Autodesk Inventor part; units mm, degrees
ref_plane "YZ Plane" through (0, 0, 0) normal (1, 0, 0) x (0, 1, 0)
ref_plane "XZ Plane" through (0, 0, 0) normal (0, 1, 0) x (-1, 0, 0)
ref_plane "XY Plane" through (0, 0, 0) normal (0, 0, 1) x (1, 0, 0)
sketch "Sketch1" plane through (0, 0, 0) normal (0, 1, 0) x (-1, 0, 0)
  circle A0 centre (0, 0) radius 84.75
  dimension "d0" = 169.5
extrude "Extrusion1" add sketch "Sketch1" along normal blind 15
sketch "Sketch2" plane through (0, 0, 0) normal (0, -1, 0) x (1, 0, 0)
  circle A0 centre (0, 0) radius 76
  circle A1 centre (0, 76) radius 4
  circle A2 centre (0, -76) radius 4
  circle A3 centre (0, 76) radius 2.25
  circle A4 centre (0, -76) radius 2.25
  dimension "d3" = 152
  dimension "d4" = 8
  dimension "d5" = 8
  dimension "d6" = 4.5
  dimension "d7" = 4.5
extrude "Extrusion2" cut sketch "Sketch2" against normal through all contours A3 A0 | A0 A3 | A4 A0 | A0 A4
extrude "Extrusion3" cut sketch "Sketch2" against normal blind 12 contours A1 A0 A3 | A0 A3 A1 | A2 A0 A4 | A0 A4 A2 | A3 A0 | A0 A3 | A4 A0 | A0 A4
sketch "Sketch3" plane through (0, 0, 0) normal (0, -1, 0) x (1, 0, 0)
  circle A0 centre (0, 0) radius 84.75
  circle A1 centre (0, 0) radius 20
  circle A2 centre (0, -20) radius 4
  circle A3 centre (20, 0) radius 4
  circle A4 centre (0, 20) radius 4
  circle A5 centre (-20, 0) radius 4
  line L0 (55, 55) -> (-55, 55)
  line L1 (-55, 55) -> (-55, -55)
  line L2 (-55, -55) -> (55, -55)
  line L3 (55, -55) -> (55, 55)
  line L4 (55, 55) -> (-55, -55) construction
  line L5 (-55, 55) -> (55, -55) construction
  circle A6 centre (0, 0) radius 55
  circle A7 centre (-38.8909, -38.8909) radius 4
  circle A8 centre (38.8909, -38.8909) radius 4
  circle A9 centre (38.8909, 38.8909) radius 4
  circle A10 centre (-38.8909, 38.8909) radius 4
  dimension "d12" = 40
  dimension "d13" = 8
  dimension "d16" = 360
  dimension "d21" = 110
  dimension "d22" = 110
  dimension "d23" = 110
  dimension "d24" = 8
  dimension "d25" = 8
  dimension "d26" = 8
  dimension "d27" = 8
hole "Hole1" at (38.8909, 0, -38.8909) at (38.8909, 0, 38.8909) at (-38.8909, 0, 38.8909) at (-38.8909, 0, -38.8909) direction (0, 1, 0) diameter 6.647 depth 20 tip angle 118
sketch "Sketch4" plane through (0, 0, 0) normal (0, -1, 0) x (1, 0, 0)
  circle A0 centre (0, 0) radius 47.5
  circle A1 centre (-47.5, 0) radius 2.5
  circle A2 centre (-43.8843, -18.1775) radius 2.5
  circle A3 centre (-33.5876, -33.5876) radius 2.5
  circle A4 centre (-18.1775, -43.8843) radius 2.5
  circle A5 centre (0, -47.5) radius 2.5
  circle A6 centre (18.1775, -43.8843) radius 2.5
  circle A7 centre (33.5876, -33.5876) radius 2.5
  circle A8 centre (43.8843, -18.1775) radius 2.5
  circle A9 centre (47.5, 0) radius 2.5
  circle A10 centre (43.8843, 18.1775) radius 2.5
  circle A11 centre (33.5876, 33.5876) radius 2.5
  circle A12 centre (18.1775, 43.8843) radius 2.5
  circle A13 centre (0, 47.5) radius 2.5
  circle A14 centre (-18.1775, 43.8843) radius 2.5
  circle A15 centre (-33.5876, 33.5876) radius 2.5
  circle A16 centre (-43.8843, 18.1775) radius 2.5
  dimension "d35" = 95
  dimension "d36" = 5
  dimension "d39" = 360
hole "Hole2" at (43.8843, 0, 18.1775) at (-43.8843, 0, -18.1775) direction (0, 1, 0) diameter 5 end through all
sketch "Sketch5" plane through (0, 15, 0) normal (0, 1, 0) x (1, 0, 0)
  circle A0 centre (0, 0) radius 84.75
hole "Hole3" at (0, 15, 0) direction (0, -1, 0) diameter 10.106 depth 32.3 tip angle 118 counterbore diameter 21 counterbore depth 13
sketch "Sketch6" plane through (0, 15, 0) normal (0, 1, 0) x (1, 0, 0)
  circle A0 centre (-38.8909, -38.8909) radius 3.3235
  circle A1 centre (-38.8909, -38.8909) radius 3.3235
  circle A2 centre (-38.8909, 38.8909) radius 3.3235
  circle A3 centre (-38.8909, 38.8909) radius 3.3235
  circle A4 centre (38.8909, 38.8909) radius 3.3235
  circle A5 centre (38.8909, 38.8909) radius 3.3235
  circle A6 centre (38.8909, -38.8909) radius 3.3235
  circle A7 centre (38.8909, -38.8909) radius 3.3235
  point P0 (0, 0)
hole "Hole4" at (-38.8909, 15, 38.8909) at (-38.8909, 15, -38.8909) at (38.8909, 15, 38.8909) at (38.8909, 15, -38.8909) direction (0, -1, 0) diameter 6.647 depth 20 tip angle 118 counterbore diameter 19 counterbore depth 9
properties part number "substrate plate"
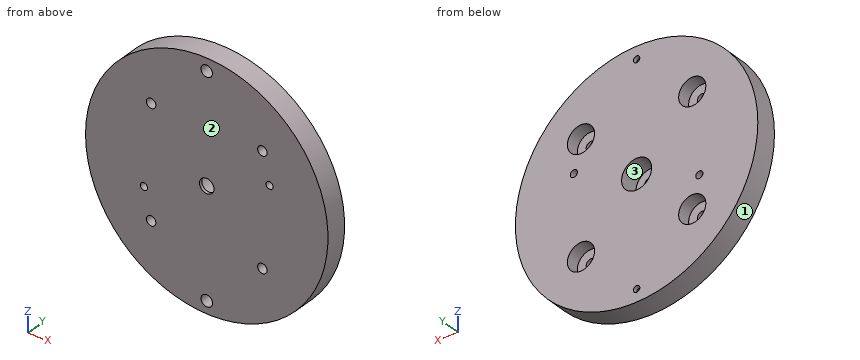
CAD build for the part. Positions are in the model's coordinates, mm. Face numbers are marked on the shaded views. Coordinates: 2 decimals unless noted, no trailing zeros. Order: outer loops, then holes, each group sorted by start corner. A loop starts at its lowest first (then second) coordinate and runs counter-clockwise, first axis right, second up. Notation, with made-up numbers: (-15.75, 2) - (0.25, 2) arc R12 cw to (0.25, 25) - close; hole circle Ø7 at (65, 69.25). An arc over 180 degrees is marked (long way). Use a Markdown table: item, result. Add a question column.
(1) Saw through at B-B (x = 0). Give the cut face in (y, z), then the cut area to 3 significant figures.
(2) Saw through at C-C (z = -76). Give the cut face in (x, y), then the cut area to 3 significant figures.
(3) Flat gauge pins, fed straight in: pin 1 (6.5 mm diameter, centred on x = 4, z = -3, fed in from +Y); pin 2 (6 mm diameter, centred on y = 10, z = -16.5, fed in from +X); pin 3 (5 mm diameter, centred on x = 0, z = -76, fed in from -Y). Where does each tip first touch, or does it go through?
(4) Pull direction X, two halves, no side cores. Call the marked faces 1, 2 and 3: +X half, -X half, draft (parallel to the pull), parting line (faces both ways), or undercut.
(5) Saw through at A-A (z = 0). Give the cut face in (x, y).
(6) Drill centre lines: line 1 along Z through (x, y) = (0, 13.5); line 2 along Z through (x, y) = (41, 10); line 3 along Z through (x, y) = (-5.5, 8.25). Where is each one in solid material? Low to high. Write a range as [from, to].
(7) Saw through at D-D (x = 31.5). Give the cut face in (y, z).
Solved:
| question | item | result |
|---|---|---|
| 1 | outline | (0, -84.75) - (15, -84.75) - (15, -78.25) - (12, -78.25) - (12, -80) - (0, -80) - close; (0, -72) - (12, -72) - (12, -73.75) - (15, -73.75) - (15, -10.5) - (2, -10.5) - (2, -5.05) - (0, -5.05) - close; (0, 5.05) - (2, 5.05) - (2, 10.5) - (15, 10.5) - (15, 73.75) - (12, 73.75) - (12, 72) - (0, 72) - close; (0, 80) - (12, 80) - (12, 78.25) - (15, 78.25) - (15, 84.75) - (0, 84.75) - close |
| 1 | area | 2,030 mm² |
| 2 | outline | (-37.5, 0) - (-4, 0) - (-4, 12) - (-2.25, 12) - (-2.25, 15) - (-37.5, 15) - close; (2.25, 12) - (4, 12) - (4, 0) - (37.5, 0) - (37.5, 15) - (2.25, 15) - close |
| 2 | area | 1,020 mm² |
| 3 | pin 1 | stops at y = 2 |
| 3 | pin 2 | stops at x = 83.67 |
| 3 | pin 3 | stops at y = 12 |
| 4 | face 1 | parting line |
| 4 | face 2 | draft |
| 4 | face 3 | undercut |
| 5 | outline | (-84.75, 0) - (-5.05, 0) - (-5.05, 2) - (-10.5, 2) - (-10.5, 15) - (-84.75, 15) - close; (5.05, 0) - (84.75, 0) - (84.75, 15) - (10.5, 15) - (10.5, 2) - (5.05, 2) - close |
| 6 | line 1 | z = [-84.75, -78.25], [-73.75, -10.5], [10.5, 73.75], [78.25, 84.75] |
| 6 | line 2 | z = [-74.17, -48.15], [-29.63, 29.63], [48.15, 74.17] |
| 6 | line 3 | z = [-84.57, -8.94], [8.94, 84.57] |
| 7 | outline | (0, -78.68) - (15, -78.68) - (15, -44.86) - (6, -44.86) - (6, -32.92) - (15, -32.92) - (15, 32.92) - (6, 32.92) - (6, 44.86) - (15, 44.86) - (15, 78.68) - (0, 78.68) - close |
